from build123d import *

# Parameters (mm, degrees)
SKETCH_W        = 55
SKETCH_H        = 75.8
PAD_DEPTH       = 3.6
SKETCH001_W     = 51.76
SKETCH001_H     = 74.18
PAD001_DEPTH    = 5
POCKET_DEPTH    = 7
SKETCH003_R     = 2
PAD002_DEPTH    = 7.25
SKETCH004_W     = 10
SKETCH004_H     = 2.5
POCKET001_DEPTH = 1
SKETCH005_W     = 10
SKETCH005_H     = 2.5
POCKET002_DEPTH = 1
POCKET003_DEPTH = 2.3
SKETCH007_R     = 1.6
POCKET004_DEPTH = 6.551
CHAMFER_SIZE    = 5
CHAMFER001_SIZE = 2
CHAMFER002_SIZE = 1
CHAMFER003_SIZE = 3
CHAMFER004_SIZE = 0.5
CHAMFER005_SIZE = 1
CHAMFER006_SIZE = 3
CHAMFER007_SIZE = 1
CHAMFER008_SIZE = 1


with BuildPart() as part:
    # Sketch → Pad (new body)
    with BuildSketch(Plane.XY):
        with Locations((27.5, 37.9)):
            Rectangle(SKETCH_W, SKETCH_H)
    extrude(amount=PAD_DEPTH)

    # Sketch001 → Pad001 (new body)
    with BuildSketch(Plane.XY.offset(3.6)):
        with Locations((27.5, 37.09)):
            Rectangle(SKETCH001_W, SKETCH001_H)
    extrude(amount=PAD001_DEPTH)

    # Sketch002 → Pocket (cut)
    with BuildSketch(Plane.XY.offset(8.6)):
        Polygon((18.22, 1.6), (3.22, 1.6), (3.22, 72.58), (51.78, 72.58), (51.78, 1.6), (36.78, 1.6), (36.78, 14.1), (18.22, 14.1), align=None)
    extrude(amount=-POCKET_DEPTH, mode=Mode.SUBTRACT)

    # Sketch003 → Pad002 (new body)
    with BuildSketch(Plane.XY.offset(1.6)):
        with Locations((10.72, 52.58)):
            Circle(SKETCH003_R)
        with Locations((44.28, 52.58)):
            Circle(SKETCH003_R)
        with Locations((18.22, 18.6)):
            Circle(SKETCH003_R)
        with Locations((36.78, 18.6)):
            Circle(SKETCH003_R)
    extrude(amount=PAD002_DEPTH)

    # Sketch004 → Pocket001 (cut)
    with BuildSketch(Plane.YZ.offset(53.38)):
        with Locations((19, 5.35)):
            Rectangle(SKETCH004_W, SKETCH004_H)
        with Locations((57.5, 5.35)):
            Rectangle(SKETCH004_W, SKETCH004_H)
    extrude(amount=-POCKET001_DEPTH, mode=Mode.SUBTRACT)

    # Sketch005 → Pocket002 (cut)
    with BuildSketch(Plane(origin=(1.62, 0, 0), x_dir=(0, -1, 0), z_dir=(-1, 0, 0))):
        with Locations((-57.5, 5.35)):
            Rectangle(SKETCH005_W, SKETCH005_H)
        with Locations((-19, 5.35)):
            Rectangle(SKETCH005_W, SKETCH005_H)
    extrude(amount=-POCKET002_DEPTH, mode=Mode.SUBTRACT)

    # Sketch006 → Pocket003 (cut)
    with BuildSketch(Plane(origin=(0, 0, 0), x_dir=(1, 0, 0), z_dir=(0, 0, -1))):
        with BuildLine():
            Line((22, 0), (33, 0))
            Line((33, 0), (33, -5.500002))
            ThreePointArc((27.500001, -11), (31.389087, -9.389088), (33, -5.500002))
            Line((27.500001, -11), (27.499999, -11))
            ThreePointArc((22, -5.500002), (23.610913, -9.389088), (27.499999, -11))
            Line((22, -5.500002), (22, 0))
        make_face()
    extrude(amount=-POCKET003_DEPTH, mode=Mode.SUBTRACT)

    # Sketch007 → Pocket004 (cut, through all)
    with BuildSketch(Plane(origin=(0, 0, 2.3), x_dir=(1, 0, 0), z_dir=(0, 0, -1))):
        with Locations((27.5, -5.5)):
            Circle(SKETCH007_R)
    extrude(amount=-POCKET004_DEPTH, mode=Mode.SUBTRACT)

    # Chamfer
    chamfer_edges = [part.edges().sort_by_distance(p)[0] for p in [
        (18.22, 14.1, 5.1),
        (36.78, 14.1, 5.1),
    ]]
    chamfer(chamfer_edges, length=CHAMFER_SIZE)

    # Chamfer001
    chamfer001_edges = [part.edges().sort_by_distance(p)[0] for p in [
        (3.22, 72.58, 5.1),
        (51.78, 72.58, 5.1),
    ]]
    chamfer(chamfer001_edges, length=CHAMFER001_SIZE)

    # Chamfer002
    chamfer002_edges = [part.edges().sort_by_distance(p)[0] for p in [
        (3.22, 36.09, 1.6),
        (4.22, 71.58, 1.6),
        (10.72, 1.6, 1.6),
        (27.5, 72.58, 1.6),
        (18.22, 5.35, 1.6),
        (50.78, 71.58, 1.6),
        (20.72, 11.6, 1.6),
        (51.78, 36.09, 1.6),
        (27.5, 14.1, 1.6),
        (44.28, 1.6, 1.6),
        (34.28, 11.6, 1.6),
        (36.78, 5.35, 1.6),
        (8.72, 52.58, 1.6),
        (42.28, 52.58, 1.6),
        (34.78, 18.6, 1.6),
        (16.22, 18.6, 1.6),
    ]]
    chamfer(chamfer002_edges, length=CHAMFER002_SIZE)

    # Chamfer003
    chamfer003_edges = [part.edges().sort_by_distance(p)[0] for p in [
        (53.38, 74.18, 6.1),
        (1.62, 74.18, 6.1),
    ]]
    chamfer(chamfer003_edges, length=CHAMFER003_SIZE)

    # Chamfer004
    chamfer004_edges = [part.edges().sort_by_distance(p)[0] for p in [
        (1.62, 35.59, 8.6),
        (3.12, 72.68, 8.6),
        (27.5, 0, 8.6),
        (27.5, 74.18, 8.6),
        (53.38, 35.59, 8.6),
        (51.88, 72.68, 8.6),
        (51.78, 36.09, 8.6),
        (50.78, 71.58, 8.6),
        (44.28, 1.6, 8.6),
        (27.5, 72.58, 8.6),
        (36.78, 5.35, 8.6),
        (4.22, 71.58, 8.6),
        (34.28, 11.6, 8.6),
        (3.22, 36.09, 8.6),
        (27.5, 14.1, 8.6),
        (10.72, 1.6, 8.6),
        (20.72, 11.6, 8.6),
        (18.22, 5.35, 8.6),
        (25.9, 5.5, 8.6),
    ]]
    chamfer(chamfer004_edges, length=CHAMFER004_SIZE)

    # Chamfer005
    chamfer005_edges = [part.edges().sort_by_distance(p)[0] for p in [
        (25.9, 5.5, 2.3),
    ]]
    chamfer(chamfer005_edges, length=CHAMFER005_SIZE)

    # Chamfer006
    chamfer006_edges = [part.edges().sort_by_distance(p)[0] for p in [
        (0, 75.8, 1.8),
        (55, 75.8, 1.8),
        (27.5, 75.8, 0),
        (55, 37.9, 0),
        (0, 37.9, 0),
    ]]
    chamfer(chamfer006_edges, length=CHAMFER006_SIZE)

    # Chamfer007
    chamfer007_edges = [part.edges().sort_by_distance(p)[0] for p in [
        (12.5, 0, 0),
        (42.5, 0, 0),
    ]]
    chamfer(chamfer007_edges, length=CHAMFER007_SIZE)

    # Chamfer008
    chamfer008_edges = [part.edges().sort_by_distance(p)[0] for p in [
        (23.610913, 9.389088, 0),
    ]]
    chamfer(chamfer008_edges, length=CHAMFER008_SIZE)


solid = part.part
Source: CAD feature listing. Evaluate the final solid. Frame: model axes, mm. A direction names the side the tool comes from. Round coordinates to 2 decimals unless told otherwise and drop trailing zeros. Write each loop counter-clockwise with the first axis right and the second up, starting at its lowest first coordinate (ties: lowest second). Pieces come first, ordered by that corner, then holes. Notation, with made-up numbers: M -0.5,62 L 14.5,62 A20 ccw 14.5,86 Z; hole C 76,-29 d3. An arc over 180 degrees is marked long. One line per item, written item: value. Start each with the question number.
Item 1: Pin query (flat end, axial travel): pin 1 (0.5 mm diameter, centred on x = 52.5, y = 55, fed in from -Z); pin 2 (4.5 mm diameter, centred on y = 5, z = 6, fed in from -X); pin 3 (3 mm diameter, centred on y = 27, z = 1, fed in from +X). Return the tip coordinate at first contact, or that it passes through.
Item 2: Set-up query: faces 4 (the cylindrical face through (38.627, 17.834, 5.681)), 5 (the flat face through (51.9, 72.66, 5.82)), 6 (the flat face through (27, 74.18, 6)). Return all of +Z, -Z, +X, -X, +Y, -Y with unobstructed straight access to the full face (end or side cutting, diameter ignored); none if empty.
Item 3: Mould query, pull axis X, two halves, no side actions, for faces 1 (the flat face through (2.62, 19, 5)), 2 (the flat face through (3.22, 36, 5)), 3 (the flat face through (27, 75, 3.6)). Classes: pulls with the +X half, pulls with the -X half, needs draft (parallel to the pull), parting line crosses it, or undercut.
Item 4: Section query B-B (y = 35). Return the cut outline in (x, z), plus the area to 3 significant figures.
Item 5: Ray query, L1, parallel to Y at x = 27.5, z = 5.85; L2, parallel to X at y = 5.5, z = 4.65; L3, parallel to X at y = 61, z = 3.25. Return the intervals inside material, ascending. Write a range as from..to.
Item 6: Section query A-A (x = 44.28). Return the cut outline in (y, z).
Result set:
1. pin 1: stops at z = 0.25
1. pin 2: stops at x = 1.62
1. pin 3: stops at x = 54.5
2. face 4: +Z
2. face 5: +Z, +X, +Y
2. face 6: +Z, +X, -X, +Y
3. face 1: pulls with the -X half
3. face 2: undercut
3. face 3: needs draft
4. outline: M 0,3 L 3,0 L 52,0 L 55,3 L 55,3.6 L 53.38,3.6 L 53.38,8.1 L 52.88,8.6 L 52.28,8.6 L 51.78,8.1 L 51.78,2.6 L 50.78,1.6 L 4.22,1.6 L 3.22,2.6 L 3.22,8.1 L 2.72,8.6 L 2.12,8.6 L 1.62,8.1 L 1.62,3.6 L 0,3.6 Z
4. area: 108 mm²
5. L1: y = 0..3.9, 7.1..14.1, 72.58..74.18
5. L2: x = 1.62..3.22, 18.22..25.9, 29.1..36.78, 51.78..53.38
5. L3: x = 0..3.22, 51.78..55
6. outline: M 0,1 L 1,0 L 72.8,0 L 75.8,3 L 75.8,3.6 L 74.18,3.6 L 74.18,8.1 L 73.68,8.6 L 73.08,8.6 L 72.58,8.1 L 72.58,2.6 L 71.58,1.6 L 55.58,1.6 L 54.58,2.6 L 54.58,8.85 L 50.58,8.85 L 50.58,2.6 L 49.58,1.6 L 2.6,1.6 L 1.6,2.6 L 1.6,8.1 L 1.1,8.6 L 0.5,8.6 L 0,8.1 Z
